Geometry: final body of the model. Coordinates: model frame, mm. Face numbers are marked on the shaded views. A direction names the side the tool comes from. Round coordinates to 2 decimals unless told otherwise and drop trailing zeros. Loops run counter-clockwise (first coordinate to the right, second up) from the corner with the lowest first, then second, coordinate; pieces in that order, holes last. Notation, with made-up numbers: (84, -23.5) -> (93, -23.5) arc R7 ccw to (93, -12.5) -> close; hole circle Ø5 at (-27, 79.25). An arc over 180 degrees is marked (long way). Answer in a Markdown table with one row per item.
```python
from build123d import *

# Parameters (mm, degrees)
BOSS_EXTRUDE1_DEPTH     = 50
SKETCH3_W               = 40
SKETCH3_H               = 20
CUT_EXTRUDE1_DEPTH      = 8
BOSS_EXTRUDE2_REACH     = 102
SKETCH4_R               = 10
SKETCH6_R               = 9
CUT_EXTRUDE2_DEPTH      = 141
CUT_EXTRUDE2_DEPTH_BACK = 1


with BuildPart() as part:
    # Sketch1 → Boss-Extrude1 (new body)
    with BuildSketch(Plane.XY):
        with BuildLine():
            Line((80, 90), (80, -10))
            Line((80, -10), (-10, -10))
            Line((-10, -10), (-10, 90))
            ThreePointArc((-10, 90), (35, 135), (80, 90))
        make_face()
        with BuildLine():
            Line((0, 90), (0, 0))
            Line((0, 0), (70, 0))
            Line((70, 0), (70, 90))
            ThreePointArc((70, 90), (35, 125), (0, 90))
        make_face(mode=Mode.SUBTRACT)
    extrude(amount=BOSS_EXTRUDE1_DEPTH)

    # Sketch3 → Cut-Extrude1 (cut)
    with BuildSketch(Plane(origin=(0, 135, 0), x_dir=(1, 0, 0), z_dir=(0, 1, 0))):
        with Locations((35, -25)):
            Rectangle(SKETCH3_W, SKETCH3_H)
    extrude(amount=-CUT_EXTRUDE1_DEPTH, mode=Mode.SUBTRACT)

    # Sketch4 → Boss-Extrude2 (add, up to next)
    with BuildSketch(Plane(origin=(0, 90, 0), x_dir=(1, 0, 0), z_dir=(0, 1, 0)), mode=Mode.PRIVATE) as boss_extrude2_sk1:
        with Locations((35, -25)):
            Circle(SKETCH4_R)
    boss_extrude2_tool1 = extrude(boss_extrude2_sk1.sketch, amount=-BOSS_EXTRUDE2_REACH, mode=Mode.PRIVATE) - part.part
    add(boss_extrude2_tool1.solids().sort_by_distance((35, 90, 25))[0])

    # Sketch6 → Cut-Extrude2 (cut, two sides)
    with BuildSketch(Plane.ZY.offset(-130)) as cut_extrude2_sk:
        with Locations((25, 50)):
            Circle(SKETCH6_R)
    extrude(amount=CUT_EXTRUDE2_DEPTH, mode=Mode.SUBTRACT)
    extrude(cut_extrude2_sk.sketch, amount=-CUT_EXTRUDE2_DEPTH_BACK, mode=Mode.SUBTRACT)


solid = part.part
```
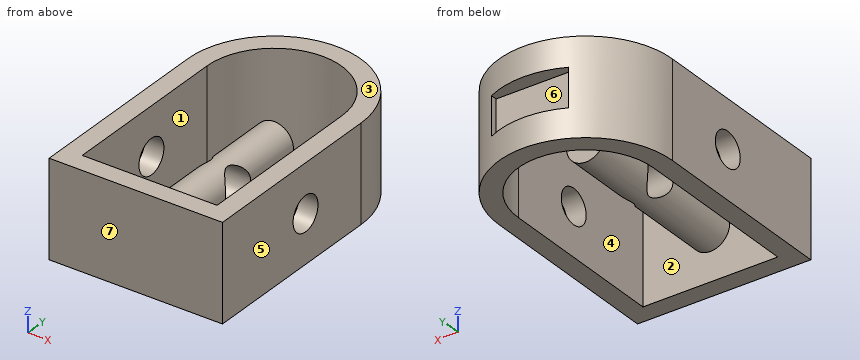
Item 1: Reachability of the marked faces 1, 2 and 3 from +Z, -Z, +X, -X, +Y, -Y: full face, straight path, thin tool, end or side. Return the list, or none.
Answer:
| item | result |
|---|---|
| face 1 | +Z, -Z |
| face 2 | none |
| face 3 | +Z, +X, -X, +Y, -Y |
Item 2: Pin query (flat end, axial travel): pin 1 Ø5 at (x, z) = (31, 21.5) entering from +Y; pin 2 Ø11 at (y, z) = (50, 25) entering from +X; pin 3 Ø3.5 at (y, z) = (129.5, 24.5) entering from +X; pin 4 Ø1 at (x, y) = (40.5, 25) entering from -Z. Return the tip coordinate at first contact, or that it passes through.
Answer:
| item | result |
|---|---|
| pin 1 | stops at y = 127 |
| pin 2 | passes through |
| pin 3 | stops at x = 59.49 |
| pin 4 | stops at z = 16.34 |
Item 3: Cut plane C-C (y = 77). Output: boundary loops of the cut face in (x, z).
Answer:
| item | result |
|---|---|
| outline | (-10, 0) -> (0, 0) -> (0, 50) -> (-10, 50) -> close; circle Ø20 at (35, 25); (70, 0) -> (80, 0) -> (80, 50) -> (70, 50) -> close |
Item 4: Cut plane D-D (z = 36.5). Output: boundary loops of the cut face in (x, y), then the cut area to 3 significant figures.
Answer:
| item | result |
|---|---|
| outline | (-10, -10) -> (80, -10) -> (80, 90) arc R45 ccw to (-10, 90) -> close; hole (0, 0) -> (70, 0) -> (70, 90) arc R35 ccw to (0, 90) -> close |
| area | 3,960 mm² |
Item 5: Cut plane B-B (z = 25). Output: boundary loops of the cut face in (x, y), then the cut area to 3 significant figures.
Answer:
| item | result |
|---|---|
| outline | (-10, -10) -> (80, -10) -> (80, 41) -> (70, 41) -> (70, 0) -> (45, 0) -> (45, 41) -> (25, 41) -> (25, 0) -> (0, 0) -> (0, 41) -> (-10, 41) -> close; (-10, 59) -> (0, 59) -> (0, 90) arc R35 cw to (70, 90) -> (70, 59) -> (80, 59) -> (80, 90) arc R45 ccw to (55, 130.31) -> (55, 127) -> (15, 127) -> (15, 130.31) arc R45 ccw to (-10, 90) -> close; (25, 59) -> (45, 59) -> (45, 90) -> (25, 90) -> close |
| area | 4,780 mm² |
Item 6: Cut plane A-A (x = 35). Output: boundary loops of the cut face in (y, z), then the cut area to 3 significant figures.
Answer:
| item | result |
|---|---|
| outline | (-10, 0) -> (0, 0) -> (0, 15) -> (90, 15) -> (90, 35) -> (0, 35) -> (0, 50) -> (-10, 50) -> close; (125, 0) -> (135, 0) -> (135, 15) -> (127, 15) -> (127, 35) -> (135, 35) -> (135, 50) -> (125, 50) -> close; hole circle Ø18 at (50, 25) |
| area | 2,390 mm² |
Item 7: Draft query along Y for the marked faces 4, 5, 6 and 7. Return one class per face: pulls with the +Y half, pulls with the -Y half, needs draft (parallel to the pull), parting line crosses it, or undercut.
Answer:
| item | result |
|---|---|
| face 4 | undercut |
| face 5 | needs draft |
| face 6 | pulls with the +Y half |
| face 7 | pulls with the -Y half |
Item 8: Line query: probe 1 along X at (y, z) = (42, 3); probe 2 along Z at (x, y) = (74, 50); probe 3 along X at (y, z) = (54, 16). Output: solid intervals per line, ascending. Write a range as [from, to].
Answer:
| item | result |
|---|---|
| probe 1 | x = [-10, 0], [70, 80] |
| probe 2 | z = [0, 16], [34, 50] |
| probe 3 | x = [-10, 0], [30.64, 39.36], [70, 80] |
